```python
from build123d import *

# Parameters (mm, degrees)
SKETCH1_R           = 3.175
BOSS_EXTRUDE1_DEPTH = 12.7
BOSS_EXTRUDE2_DEPTH = 19.05
CUT_EXTRUDE2_DEPTH  = 30.48
BOSS_EXTRUDE7_DEPTH = 25.4
BOSS_EXTRUDE8_DEPTH = 19.05
CUT_EXTRUDE3_DEPTH  = 41.148
BOSS_EXTRUDE9_DEPTH = 25.4


with BuildPart() as part:
    # Sketch1 → Boss-Extrude1 (new body)
    with BuildSketch(Plane.XY):
        with BuildLine():
            Line((299.870251741, -63.185614448), (503.070251741, -63.185614448))
            ThreePointArc((503.070251741, -63.185614448), (518.945251741, -79.060614448), (503.070251741, -94.935614448))
            Line((503.070251741, -94.935614448), (299.870251741, -94.935614448))
            ThreePointArc((299.870251741, -94.935614448), (283.995251741, -79.060614448), (299.870251741, -63.185614448))
        make_face()
        with Locations((299.870251741, -79.060614448)):
            Circle(SKETCH1_R, mode=Mode.SUBTRACT)
        with Locations((503.070251741, -79.060614448)):
            Circle(SKETCH1_R, mode=Mode.SUBTRACT)
    extrude(amount=BOSS_EXTRUDE1_DEPTH)

    # Sketch2 → Boss-Extrude2 (add)
    with BuildSketch(Plane(origin=(0, 0, 0), x_dir=(-1, 0, 0), z_dir=(0, 0, -1))):
        with BuildLine():
            Line((-477.670251741, -66.360614448), (-477.670251741, -91.760614448))
            Line((-477.670251741, -91.760614448), (-513.230251741, -91.760614448))
            ThreePointArc((-513.230251741, -91.760614448), (-515.026302965, -91.016665672), (-515.770251741, -89.220614448))
            Line((-515.770251741, -89.220614448), (-515.770251741, -68.900614448))
            ThreePointArc((-515.770251741, -68.900614448), (-515.026302965, -67.104563223), (-513.230251741, -66.360614448))
            Line((-513.230251741, -66.360614448), (-477.670251741, -66.360614448))
        make_face()
    extrude(amount=BOSS_EXTRUDE2_DEPTH)

    # Sketch6 → Cut-Extrude2 (cut)
    with BuildSketch(Plane.XZ.offset(91.760614448)):
        with BuildLine():
            Line((499.246061033, 0), (515.770251741, 0))
            Line((515.770251741, 0), (515.770251741, -14.733462418))
            Line((515.770251741, -14.733462418), (491.640251741, -14.733462418))
            ThreePointArc((491.640251741, -14.733462418), (485.287193282, -8.73432293), (485.036934778, 0))
            Line((485.036934778, 0), (488.908392954, 0))
            Line((488.908392954, 0), (499.246061033, 0))
        make_face()
    extrude(amount=-CUT_EXTRUDE2_DEPTH, mode=Mode.SUBTRACT)

    # Sketch4 → Boss-Extrude7 (add)
    with BuildSketch(Plane.XZ.offset(91.760614448)):
        Polygon((477.670251741, -19.05), (450.464032212, 0), (477.670251741, 0), align=None)
    extrude(amount=-BOSS_EXTRUDE7_DEPTH)

    # Sketch7 → Boss-Extrude8 (add)
    with BuildSketch(Plane.XY.offset(12.7)):
        with BuildLine():
            Line((310.030251741, -66.360614448), (312.570251741, -66.360614448))
            Line((312.570251741, -66.360614448), (322.730251741, -66.360614448))
            Line((322.730251741, -66.360614448), (322.730251741, -91.760614448))
            Line((322.730251741, -91.760614448), (310.030251741, -91.760614448))
            Line((310.030251741, -91.760614448), (289.710251741, -91.760614448))
            ThreePointArc((289.710251741, -91.760614448), (287.914200517, -91.016665672), (287.170251741, -89.220614448))
            Line((287.170251741, -89.220614448), (287.170251741, -68.900614448))
            ThreePointArc((287.170251741, -68.900614448), (287.914200517, -67.104563223), (289.710251741, -66.360614448))
            Line((289.710251741, -66.360614448), (310.030251741, -66.360614448))
        make_face()
    extrude(amount=BOSS_EXTRUDE8_DEPTH)

    # Sketch8 → Cut-Extrude3 (cut)
    with BuildSketch(Plane(origin=(0, -66.360614448, 0), x_dir=(1, 0, 0), z_dir=(0, 1, 0))):
        with BuildLine():
            Line((287.170251741, -12.7), (317.904251741, -12.7))
            ThreePointArc((317.904251741, -12.7), (317.648023156, -21.431345807), (311.300251741, -27.432))
            Line((311.300251741, -27.432), (287.170251741, -27.432))
            Line((287.170251741, -27.432), (287.170251741, -12.7))
        make_face()
    extrude(amount=-CUT_EXTRUDE3_DEPTH, mode=Mode.SUBTRACT)

    # Sketch9 → Boss-Extrude9 (add)
    with BuildSketch(Plane(origin=(0, -66.360614448, 0), x_dir=(1, 0, 0), z_dir=(0, 1, 0))):
        Polygon((322.730251741, -31.75), (349.936471269, -12.7), (322.730251741, -12.7), align=None)
    extrude(amount=-BOSS_EXTRUDE9_DEPTH)


solid = part.part
```
Part model, mm, in its own coordinate system. A direction names the side the tool comes from. Round coordinates to 2 decimals unless told otherwise and drop trailing zeros. Write each loop counter-clockwise with the first axis right and the second up, starting at its lowest first coordinate (ties: lowest second). Pieces come first, ordered by that corner, then holes. Notation, with made-up numbers: (47.25, 37) -> (98.25, 37) arc R15 ccw to (98.25, 45) -> close; hole circle Ø6 at (65, 29.25). An arc over 180 degrees is marked (long way). Return JSON: item names as keys, results as strings. Group by question number.
Q1. Probe L1, parallel to Z at x = 497.5, y = -69; L2, parallel to Z at x = 432, y = -70; L3, parallel to Z at x = 478.5, y = -86.5. List the from-to ranges inside material, lowest first. Write a range as [from, to].
Q2. Saw through at C-C on z = 6. Write the cut outline in (x, y) (3 decimals), plus the area to 3 significant figures.
Q3. Saw through at B-B on y = -71. Write the cut outline in (x, z), plus the area to 3 significant figures.
Q4. Mould opens along Z. For faces 5 (the flat face through (305, -79, 31.75)), 6 (the cylindrical face through (518.94, -78.71, 6.26)), 7 (the flat face through (299, -79, 27.432)), 8 (the cylindrical face through (317.699, -78.883, 21.317)) say: pulls with the +Z half, pulls with the -Z half, needs draft (parallel to the pull), parting line crosses it, or undercut.
Q5. Saw through at A-A on x = 333. Write the cut outline in (y, z), plus the area to 3 significant figures.
Q6. Which spindle directions (+Z, -Z, +X, -X, +Y, -Y) get a long thin tool onto all of the face, cutting with end or side? Do faces 1 (the flat face through (319, -66.361, 22)), 2 (the cylindrical face through (296.7, -78.9, 6.3)), 3 (the flat face through (482, -66.361, -9)), 4 (the flat face through (515.77, -79, -17)). Say none if no direction does.
Q7. Saw through at D-D on z = 22. Write the cut outline in (x, y), plus the area to 3 significant figures.
Q8. Pin check, flat tips, straight feed: pin 1 (21 mm diameter, centred on x = 310, z = 26.5, fed in from -Y); pin 2 (12 mm diameter, centred on x = 344.5, z = 17.5, fed in from +Y); pin 3 (1.3 mm diameter, centred on y = -84, z = -16, fed in from +X); pin 4 (5.5 mm diameter, centred on x = 468.5, z = -13, fed in from +Y). Stop position of each tip, or through.
Answer:
{
 "1": {"L1": "[-19.05, -14.73], [0, 12.7]", "L2": "[0, 12.7]", "L3": "[-19.05, 12.7]"},
 "2": {"outline": "(299.87, -94.936) -> (503.07, -94.936) arc R15.875 ccw to (503.07, -63.186) -> (299.87, -63.186) arc R15.875 ccw to start; hole circle Ø6.35 at (299.87, -79.061); hole circle Ø6.35 at (503.07, -79.061)", "area": "7,180 mm2"},
 "3": {"outline": "(286.19, 0) -> (450.46, 0) -> (477.67, -19.05) -> (515.77, -19.05) -> (515.77, -14.73) -> (491.64, -14.73) arc R11.42 cw to (485.04, 0) -> (516.75, 0) -> (516.75, 12.7) -> (349.94, 12.7) -> (322.73, 31.75) -> (287.17, 31.75) -> (287.17, 27.43) -> (311.3, 27.43) arc R11.43 cw to (317.9, 12.7) -> (286.19, 12.7) -> close", "area": "3,970 mm2"},
 "4": {"face 5": "pulls with the +Z half", "face 6": "needs draft", "face 7": "undercut", "face 8": "undercut"},
 "5": {"outline": "(-94.94, 0) -> (-63.19, 0) -> (-63.19, 12.7) -> (-66.36, 12.7) -> (-66.36, 24.56) -> (-91.76, 24.56) -> (-91.76, 12.7) -> (-94.94, 12.7) -> close", "area": "704 mm2"},
 "6": {"face 1": "+Z, +X, -X, +Y", "face 2": "-Z", "face 3": "-Z, +X, -X, +Y", "face 4": "-Z, +X, +Y, -Y"},
 "7": {"outline": "(317.37, -91.76) -> (336.65, -91.76) -> (336.65, -66.36) -> (317.37, -66.36) -> close", "area": "490 mm2"},
 "8": {"pin 1": "y = -91.76", "pin 2": "y = -63.19", "pin 3": "x = 515.77", "pin 4": "y = -66.36"}
}
